```python
from build123d import *

# Parameters (mm, degrees)
EXTRUDE_11098_DEPTH         = 26
FILLET_11147_R              = 2.5
SHELL_11558_T               = 2.4
SKETCH_12788_W              = 77
SKETCH_12788_H              = 26
CUT_EXTRUDE_13245_DEPTH     = 1.2
CUT_EXTRUDE_START           = -2.4
CUT_EXTRUDE_14712_OUTLINE_W = 8
CUT_EXTRUDE_14712_OUTLINE_H = 7
CUT_EXTRUDE_14712_DEPTH     = 2.4
CUT_EXTRUDE_START_2         = -3
CUT_EXTRUDE_16699_OUTLINE_W = 11
CUT_EXTRUDE_16699_OUTLINE_H = 9
CUT_EXTRUDE_16699_OUTLINE_R = 3
CUT_EXTRUDE_16699_DEPTH     = 4
SKETCH_16755_R              = 1.4
CUT_EXTRUDE_17028_DEPTH     = 3
SKETCH_17076_R              = 1.4
CUT_EXTRUDE_17283_DEPTH     = 3
CHAMFER_17332_SIZE          = 0.8
FILLET_1_R                  = 0.4
SKETCH_19008_R              = 2.5
CUT_EXTRUDE_19107_DEPTH     = 100


with BuildPart() as part:
    # Extrude 11098: read off the stored shape, not the designer's step
    # Extrude 11098 outline → Extrude 11098 (new body)
    with BuildSketch(Plane.XY):
        with BuildLine():
            ThreePointArc((50, 154.142813358), (8.283821468, 161.837527205), (-34, 158.442440368))
            Line((-34, 158.442440368), (-34, 91.699111876))
            ThreePointArc((-34, 91.699111876), (8.866783155, 97.3966492), (50, 84.051931084))
            Line((50, 84.051931084), (50, 154.142813358))
        make_face()
    extrude(amount=EXTRUDE_11098_DEPTH)

    # Fillet 11147
    fillet_11147_edges = [part.edges().sort_by_distance(p)[0] for p in [
        (8.866783155, 97.3966492, 26),
        (50, 119.097372221, 26),
        (8.283821468, 161.837527205, 26),
        (50, 154.142813358, 13),
        (50, 84.051931084, 13),
        (-34, 91.699111876, 13),
        (-34, 158.442440368, 13),
        (-34, 125.070776122, 26),
    ]]
    fillet(fillet_11147_edges, radius=FILLET_11147_R)

    # Shell 11558
    shell_11558_openings = [part.faces().sort_by_distance(p)[0] for p in [
        (8.321154323, 127.154130668, 0),
    ]]
    offset(amount=SHELL_11558_T, openings=shell_11558_openings, kind=Kind.INTERSECTION)

    # Cut-Extrude 12697: read off the stored shape, not the designer's step
    # Cut-Extrude 12697: loft between two sections, ruled curve by curve
    cut_extrude_12697_from = [
        Edge.make_line((-24.6, 126.4, 26), (40.6, 126.4, 26)),
        Edge.make_line((-24.6, 141.6, 26), (-24.6, 126.4, 26)),
        Edge.make_line((40.6, 141.6, 26), (-24.6, 141.6, 26)),
        Edge.make_line((40.6, 126.4, 26), (40.6, 141.6, 26)),
    ]
    cut_extrude_12697_to = [
        Edge.make_line((-27, 124, 28.4), (43, 124, 28.4)),
        Edge.make_line((-27, 144, 28.4), (-27, 124, 28.4)),
        Edge.make_line((43, 144, 28.4), (-27, 144, 28.4)),
        Edge.make_line((43, 124, 28.4), (43, 144, 28.4)),
    ]
    cut_extrude_12697 = Solid(Shell([*[Face.make_surface_from_curves(cut_extrude_12697_from[k], cut_extrude_12697_to[k]) for k in range(4)], Face(Wire(cut_extrude_12697_from)), Face(Wire(cut_extrude_12697_to))]))
    add(cut_extrude_12697, mode=Mode.SUBTRACT)

    # Sketch 12788 → Cut-Extrude 13245 (cut)
    with BuildSketch(Plane(origin=(0, 0, 26), x_dir=(-1, 0, 0), z_dir=(0, 0, -1))):
        with Locations((-8, 134)):
            Rectangle(SKETCH_12788_W, SKETCH_12788_H)
    extrude(amount=-CUT_EXTRUDE_13245_DEPTH, mode=Mode.SUBTRACT)

    # Cut-Extrude 14712: read off the stored shape, not the designer's step
    # Cut-Extrude 14712 outline → Cut-Extrude 14712 (cut)
    with BuildSketch(Plane.XY.offset(28.4).offset(CUT_EXTRUDE_START)):
        with Locations((26.004631823, 111.792348678)):
            Rectangle(CUT_EXTRUDE_14712_OUTLINE_W, CUT_EXTRUDE_14712_OUTLINE_H)
        with Locations((14.004631823, 111.792348678)):
            Rectangle(CUT_EXTRUDE_14712_OUTLINE_W, CUT_EXTRUDE_14712_OUTLINE_H)
        with Locations((2.004631823, 111.792348678)):
            Rectangle(CUT_EXTRUDE_14712_OUTLINE_W, CUT_EXTRUDE_14712_OUTLINE_H)
        with Locations((-9.995368177, 111.792348678)):
            Rectangle(CUT_EXTRUDE_14712_OUTLINE_W, CUT_EXTRUDE_14712_OUTLINE_H)
    extrude(amount=CUT_EXTRUDE_14712_DEPTH, mode=Mode.SUBTRACT)

    # Cut-Extrude 16699: read off the stored shape, not the designer's step
    # Cut-Extrude 16699 outline → Cut-Extrude 16699 (cut)
    with BuildSketch(Plane(origin=(52.4, 0, 0), x_dir=(0, 0, -1), z_dir=(1, 0, 0)).offset(CUT_EXTRUDE_START_2)):
        with Locations((-11.5, 100.5)):
            Rectangle(CUT_EXTRUDE_16699_OUTLINE_W, CUT_EXTRUDE_16699_OUTLINE_H)
        with Locations((-13, 111)):
            Circle(CUT_EXTRUDE_16699_OUTLINE_R)
        Polygon((-14.3, 128.5), (-13.6, 129.7), (-11.8, 129.7), (-11.8, 135.3), (-13.6, 135.3), (-14.3, 136.5), (-15.8, 136.5), (-15.8, 128.5), align=None)
    extrude(amount=CUT_EXTRUDE_16699_DEPTH, mode=Mode.SUBTRACT)

    # Sketch 16755 → Cut-Extrude 17028 (cut)
    with BuildSketch(Plane(origin=(52.4, 0, 0), x_dir=(0, 0, -1), z_dir=(1, 0, 0))):
        with Locations(Location((-2.25, 91.438690467, 0), (0, 0, 90))):
            Circle(SKETCH_16755_R)
        with Locations(Location((-2.25, 144.314674038, 0), (0, 0, 90))):
            Circle(SKETCH_16755_R)
    extrude(amount=-CUT_EXTRUDE_17028_DEPTH, mode=Mode.SUBTRACT)

    # Sketch 17076 → Cut-Extrude 17283 (cut)
    with BuildSketch(Plane.ZY.offset(36.4).offset(CUT_EXTRUDE_START_2)):
        with Locations(Location((2.25, 103.724598888, 0), (0, 0, 270))):
            Circle(SKETCH_17076_R)
        with Locations(Location((2.25, 144.314674038, 0), (0, 0, 90))):
            Circle(SKETCH_17076_R)
    extrude(amount=CUT_EXTRUDE_17283_DEPTH, mode=Mode.SUBTRACT)

    # Chamfer 17332
    chamfer_17332_edges = [part.edges().sort_by_distance(p)[0] for p in [
        (52.4, 90.038690467, 2.25),
        (52.4, 142.914674038, 2.25),
        (-36.4, 142.914674038, 2.25),
        (-36.4, 105.124598888, 2.25),
    ]]
    chamfer(chamfer_17332_edges, length=CHAMFER_17332_SIZE)

    # Скругление1
    fillet_1_edges = [part.edges().sort_by_distance(p)[0] for p in [
        (-5.995368177, 115.292348678, 27.2),
        (-5.995368177, 108.292348678, 27.2),
        (-13.995368177, 108.292348678, 27.2),
        (-13.995368177, 115.292348678, 27.2),
        (-1.995368177, 108.292348678, 27.2),
        (-1.995368177, 115.292348678, 27.2),
        (6.004631823, 115.292348678, 27.2),
        (6.004631823, 108.292348678, 27.2),
        (10.004631823, 108.292348678, 27.2),
        (10.004631823, 115.292348678, 27.2),
        (18.004631823, 115.292348678, 27.2),
        (18.004631823, 108.292348678, 27.2),
        (22.004631823, 108.292348678, 27.2),
        (22.004631823, 115.292348678, 27.2),
        (30.004631823, 115.292348678, 27.2),
        (30.004631823, 108.292348678, 27.2),
    ]]
    fillet(fillet_1_edges, radius=FILLET_1_R)

    # Sketch 19008 → Cut-Extrude 19107 (cut)
    with BuildSketch(Plane(origin=(0, 0, 0), x_dir=(1, 0, 0), z_dir=(0, 1, 0))):
        with Locations(Location((31.62731448, -8.5, 0), (0, 0, 90))):
            Circle(SKETCH_19008_R)
    extrude(amount=CUT_EXTRUDE_19107_DEPTH, mode=Mode.SUBTRACT)


solid = part.part
```
Input: part model. Units: mm. Frame: model coordinates. A direction names the side the tool comes from. Round coordinates to 2 decimals unless told otherwise and drop trailing zeros. Write each loop counter-clockwise with the first axis right and the second up, starting at its lowest first coordinate (ties: lowest second). Pieces come first, ordered by that corner, then holes. Notation, with made-up numbers: M 72,55.25 L 104,55.25 A19 ccw 104,69.25 Z; hole C -19.5,-4 d5. An arc over 180 degrees is marked long. Write each question's results on one line, items separated by ' | '.
Q1. Section query B-B (z = 22.5). Return loops of the section in (x, y).
Results:
outline: M -36.4,95.22 A4.9 ccw -29.96,90.57 A95.4 cw 45.18,84.02 A4.9 ccw 52.4,88.34 L 52.4,152.31 A4.9 ccw 48.96,156.99 A164.45 ccw -32.47,161.21 A4.9 ccw -36.4,156.41 Z; hole M -34,95.22 A2.5 ccw -30.71,92.85 A97.8 cw 46.32,86.14 A2.5 ccw 50,88.34 L 50,152.31 A2.5 ccw 48.24,154.7 A162.05 ccw -31.99,158.86 A2.5 ccw -34,156.41 Z
Q2. Section query C-C (z = 8.5). Return loops of the section in (x, y).
Results:
outline: M -36.4,95.22 A4.9 ccw -29.96,90.57 A95.4 cw 29.13,90.84 L 29.13,93.36 A97.8 ccw -30.71,92.85 A2.5 cw -34,95.22 L -34,156.41 A2.5 cw -31.99,158.86 A162.05 cw 48.24,154.7 A2.5 cw 50,152.31 L 50,105 L 52.4,105 L 52.4,152.31 A4.9 ccw 48.96,156.99 A164.45 ccw -32.47,161.21 A4.9 ccw -36.4,156.41 Z; M 34.13,89.09 A95.4 cw 45.18,84.02 A4.9 ccw 52.4,88.34 L 52.4,96 L 50,96 L 50,88.34 A2.5 cw 46.32,86.14 A97.8 ccw 34.13,91.65 Z
Q3. Access query for faces 4 (the face through (7, 117, 26)), 5 (the face through (-36.4, 126, 12)), 6 (the face through (14, 115.292, 27)), 7 (the face through (51, 133, 15.8)). Directions: +Z, -Z, +X, -X, +Y, -Y. A direction counts if a zero-diameter tool reaches every point of the face in a straight line with its end or side. Return the directions, or none.
Results:
face 4: -Z | face 5: +Z, -Z, -X, +Y, -Y | face 6: +Z, -Z | face 7: +X
Q4. Line query: line 1 along X through (y, z) = (125, 6.5); line 2 along Z through (x, y) = (51.7, 111); line 3 along Y through (x, z) = (51.4, 13). Output: solid intervals per line, ascending.
Results:
line 1: x = -36.4 to -34, 50 to 52.4 | line 2: z = 0 to 10, 16 to 26.02 | line 3: y = 85.37 to 96, 105 to 108, 114 to 129.7, 135.3 to 155.28
Q5. Pin query (flat end, axial travel): P1, Ø8, axis at x = 31.63, z = 8.5, coming from the -Y side; P2, Ø1, axis at x = 32, z = 24, coming from the -Y side; P3, Ø1.3, axis at y = 138.5, z = 26.5, coming from the +X side. Return the tip coordinate at first contact, or that it passes through.
Results:
P1: stops at y = 88.5 | P2: stops at y = 89.71 | P3: stops at x = 51.8
Q6. Draft query along Y for faces 1 (the face through (50.811, 142.916, 2.312)), 2 (the face through (52.4, 120, 12)), 3 (the face through (49.953, 84.097, 11.914)). Return one class per face: released by +Y, released by -Y, zero draft, split by the parting line, or undercut.
Results:
face 1: undercut | face 2: zero draft | face 3: released by -Y
Q7. Section query A-A (y = 111). State how many separate pieces and enclosed holes the cut face has, and give its area (3 significant figures).
Results:
separate pieces: 6 | enclosed holes: 0 | area: 239 mm^2
